Job drawing, mm, ordinate dimensions from the low corner. One solid piece. A direction names the side the tool comes from. Give positions to 0.01 mm unless a question says otherwise; leave off trailing zeros. Write each loop counter-clockwise with the first axis right and the second up, starting at its lowest first coordinate (ties: lowest second). Pieces come first, ordered by that corner, then holes. Notation, with made-up numbers: M 57.5,71 L 62.5,71 A35 ccw 62.5,104 Z; hole C 47.25,11.25 d7. An arc over 180 degrees is marked long. Answer as CSV lines item,"result". Start each with the question number.
1) Wall check: line 1 along Y through (x, z) = (14, 17.75) (1 decimal); line 2 along Y through (x, z) = (20.5, 15); line 3 along Z through (x, y) = (14, 4). Give the ranges that are in metal, low to high. Write a range as from..to.
2) Slice it at A-A, the plane z = 14. Give the cut face in (x, y) (1 decimal).
3) Tool access for the marked faces 4, 5 and 6: list every direction of +Z, -Z, +X, -X, +Y, -Y with a clear straight run to the whole face (end or side of a thin tool).
4) Slice it at C-C, the plane y = 4. Give the cut face in (x, z) (1 decimal), plus the area to 3 significant figures.
5) Slice it at B-B, the plane x = 14. Give the cut face in (y, z) (1 decimal).
6) Slice it at D-D, the plane y = 10.75. Give the cut face in (x, z).
7) Mould opens along X. For the marked faces 1, 2 and 3 say: pulls with the +X half, pulls with the -X half, needs draft (parallel to the pull), parting line crosses it, or undercut.
8) Pin check, flat tips, straight feed: pin 1 Ø2.5 at (y, z) = (4, 14) entering from +X; pin 2 Ø5 at (x, z) = (3, 19) entering from -Y; pin 3 Ø6 at (x, y) = (18.5, 8.5) entering from -Z; pin 4 Ø2 at (x, z) = (14, 24) entering from +Y. Stop position of each tip, or through.
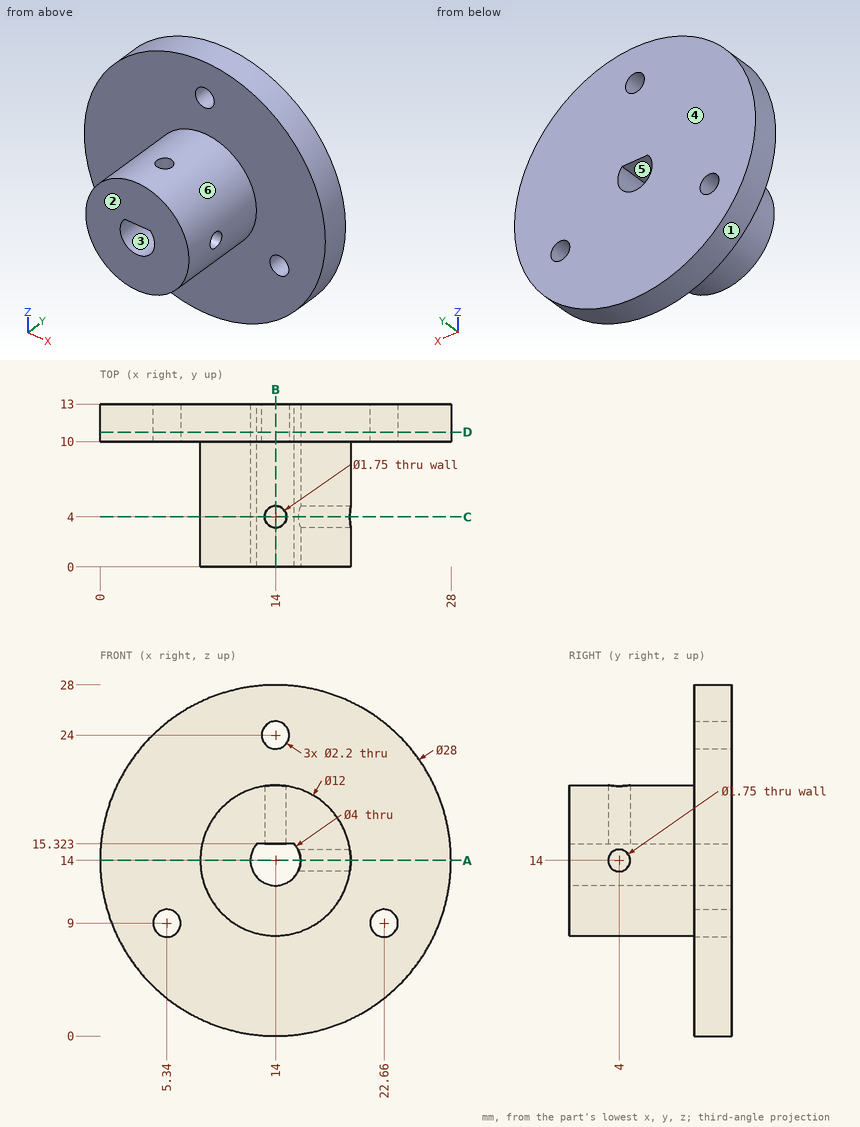
Found:
1,line 1,"0..3.1, 4.9..13"
1,line 2,"10..13"
1,line 3,"8..12"
2,outline,"M 0,10 L 8,10 L 8,0 L 12,0 L 12,13 L 0,13 Z; M 16,0 L 20,0 L 20,3.1 L 16,3.1 Z; M 16,4.9 L 20,4.9 L 20,10 L 28,10 L 28,13 L 16,13 Z"
3,face 4,"+Z, -Z, +X, -X, +Y"
3,face 5,"+Y, -Y"
3,face 6,"-Y"
4,outline,"M 12.5,15.3 L 13.1,15.3 L 13.1,19.9 A6 ccw long 19.9,13.1 L 15.8,13.1 A2 cw long Z; M 14.9,15.3 L 15.5,15.3 A2 cw 15.8,14.9 L 19.9,14.9 A6 ccw 14.9,19.9 Z"
4,area,"86.7 mm²"
5,outline,"M 0,8 L 10,8 L 10,0 L 13,0 L 13,12 L 0,12 Z; M 0,15.3 L 3.1,15.3 L 3.1,20 L 0,20 Z; M 4.9,15.3 L 13,15.3 L 13,22.9 L 10,22.9 L 10,20 L 4.9,20 Z; M 10,25.1 L 13,25.1 L 13,28 L 10,28 Z"
6,outline,"C 14,14 d28; hole C 5.34,9 d2.2; hole M 12.5,15.32 A2 ccw long 15.5,15.32 Z; hole C 14,24 d2.2; hole C 22.66,9 d2.2"
7,face 1,"parting line crosses it"
7,face 2,"needs draft"
7,face 3,"undercut"
8,pin 1,"x = 20"
8,pin 2,"y = 10"
8,pin 3,"z = 0.13"
8,pin 4,"through"
